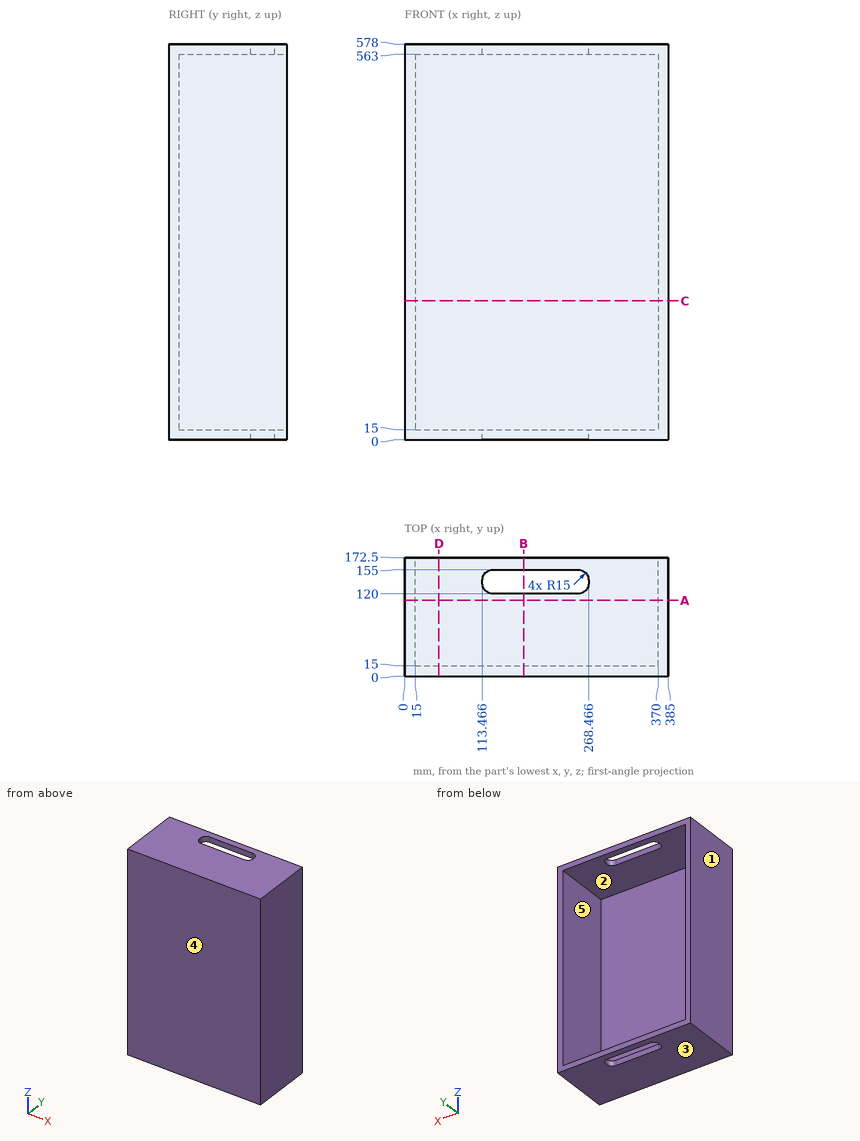
Geometry: see drawing. Coordinates: mm, zero at the bounding-box minimum. A direction names the side the tool comes from. Give positions to 0.01 mm unless a question says otherwise; leave off trailing zeros. Loops run counter-clockwise (first coordinate to the right, second up) from the corner with the lowest first, then second, coordinate; pieces in that order, holes last. Notation, with made-up numbers: (-13, 32.25) -> (29, 32.25) arc R24 cw to (29, 42.25) -> close; hole circle Ø3 at (27, -28). An arc over 180 degrees is marked (long way). Use one line per item in the form item = value.
Item 1: Pin query (flat end, axial travel): P1, Ø1, axis at x = 275, z = 204, coming from the +Y side. Return the tip coordinate at first contact, or that it passes through.
A:
P1 = 15
Item 2: Section query A-A on y = 110.5. Output: boundary loops of the cut face in (x, z), and give its area (3 significant figures).
A:
outline = (0, 0) -> (385, 0) -> (385, 578) -> (0, 578) -> close; hole (15, 15) -> (370, 15) -> (370, 563) -> (15, 563) -> close
area = 28,000 mm^2
Item 3: Section query C-C on z = 203. Output: boundary loops of the cut face in (x, y), and give its area (3 significant figures).
A:
outline = (0, 0) -> (385, 0) -> (385, 172.5) -> (370, 172.5) -> (370, 15) -> (15, 15) -> (15, 172.5) -> (0, 172.5) -> close
area = 10,500 mm^2
Item 4: Draft query along Z for the marked faces 3, 4 and 5. Return one class per face: pulls with the +Z half, pulls with the -Z half, needs draft (parallel to the pull), parting line crosses it, or undercut.
A:
face_3 = pulls with the -Z half
face_4 = needs draft
face_5 = undercut
Item 5: Line query: probe 1 along Z at (x, y) = (99, 79.5); probe 2 along X at (y, z) = (141, 183); probe 3 along Y at (x, z) = (44, 234.5). Output: solid intervals per line, ascending.
A:
probe_1 = 0 to 15, 563 to 578
probe_2 = 0 to 15, 370 to 385
probe_3 = 0 to 15
Item 6: Access query for the marked faces 1 and 2. Directions: +Z, -Z, +X, -X, +Y, -Y. A direction counts if a zero-diameter tool reaches every point of the face in a straight line with its end or side. Return the directions, or none.
A:
face_1 = +Z, -Z, -X, +Y, -Y
face_2 = +Y
Item 7: Section query B-B on x = 173.5. Output: boundary loops of the cut face in (y, z), and give its area (3 significant figures).
A:
outline = (0, 0) -> (120, 0) -> (120, 15) -> (15, 15) -> (15, 563) -> (120, 563) -> (120, 578) -> (0, 578) -> close; (155, 0) -> (172.5, 0) -> (172.5, 15) -> (155, 15) -> close; (155, 563) -> (172.5, 563) -> (172.5, 578) -> (155, 578) -> close
area = 12,300 mm^2
Item 8: Section query D-D on x = 50. Output: boundary loops of the cut face in (y, z), and give its area (3 significant figures).
A:
outline = (0, 0) -> (172.5, 0) -> (172.5, 15) -> (15, 15) -> (15, 563) -> (172.5, 563) -> (172.5, 578) -> (0, 578) -> close
area = 13,400 mm^2
